Input: part model. Units: mm. Frame: model coordinates. A direction names the side the tool comes from. Coordinates: 2 decimals unless noted, no trailing zeros. Write each loop counter-clockwise with the first axis right and the second up, starting at its lowest first coordinate (ties: lowest second). Pieces come first, ordered by that corner, then holes. Notation, with made-up numbers: (47.25, 71.5) - (90.25, 71.5) arc R19 ccw to (90.25, 101.5) - close; hole circle Ø10 at (-29, 89.5). An arc over 180 degrees is marked (long way). Use a Markdown table: item, result. Add a question column.
Q1. Pin query (flat end, axial travel): P1, Ø2, axis at x = 10.16, z = 2.5, coming from the -Y side; P2, Ø1, axis at y = -9.5, z = 1.5, coming from the +X side. Return the tip coordinate at first contact, or that it passes through.
Q2. Section query A-A (z = 2.5). Return the cut outline in (x, y), then the cut area to 3 significant figures.
Q3. Section query D-D (x = 6.8). Return the cut outline in (y, z), then the cut area to 3 significant figures.
Q4. Mould query, pull axis Y, two halves, no side actions, for faces 6 (the face through (8, -25, 2)), 7 (the face through (8, -4, 1)), 8 (the face through (3.6, -14.3, 5)), 9 (the face through (5, 0, 2)). Classes: released by +Y, released by -Y, zero draft, split by the parting line, or undercut.
Q5. Material intervals for probe 1 along Y at (x, z) = (7, 0.4); probe 2 along Z at (x, y) = (10.16, -27.6); probe 3 along X at (y, z) = (-6.5, 4), sorted ascending. Write a range as from..to.
Q6. Set-up query: faces 1 (the face through (4, -14, 2)), 2 (the face through (9.6, -2, 2)), 3 (the face through (8.54, -27.03, 1.99)), 4 (the face through (6, -29, 2)), 5 (the face through (8.5, -2.03, 2.43)). Return all of +Z, -Z, +X, -X, +Y, -Y with unobstructed straight access to the full face (end or side cutting, diameter ignored); none if empty.
Q7. Section query B-B (x = 10.16). Return the cut outline in (y, z).
Q8. Section query C-C (y = -25.75). Return the cut outline in (x, z), then the cut area to 3 significant figures.
from build123d import *

# Parameters (mm, degrees)
RESSALTO_EXTRUS_O1_DEPTH    = 5
FURO_COM_FOLGA_DE_M32_D     = 3.4
FURO_COM_FOLGA_DE_M32_DEPTH = 4
FURO_COM_FOLGA_DE_M31_D     = 3.4
FURO_COM_FOLGA_DE_M31_DEPTH = 11.25
FURO_COM_FOLGA_DE_M31_TIP   = 1.021463052


with BuildPart() as part:
    # Esboço1 → Ressalto-extrusão1 (new body)
    with BuildSketch(Plane.XY):
        Polygon((12.7, -29), (0, -29), (0, 0), (9.6, 0), (9.6, -4), (4, -4), (4, -25), (12.7, -25), align=None)
    extrude(amount=RESSALTO_EXTRUS_O1_DEPTH)

    # Furo com folga de M32
    with Locations(Plane(origin=(0, -25, 0), x_dir=(1, 0, 0), z_dir=(0, 1, 0))):
        with Locations((10.16, -2.5)):
            Hole(FURO_COM_FOLGA_DE_M32_D / 2, depth=FURO_COM_FOLGA_DE_M32_DEPTH)

    # Furo com folga de M31
    with Locations(Plane(origin=(0, 0, 0), x_dir=(1, 0, 0), z_dir=(0, 1, 0))):
        with Locations((6.8, -2.5)):
            Hole(FURO_COM_FOLGA_DE_M31_D / 2, depth=FURO_COM_FOLGA_DE_M31_DEPTH)
            with Locations((0, 0, -(FURO_COM_FOLGA_DE_M31_DEPTH + FURO_COM_FOLGA_DE_M31_TIP / 2))):  # 118° drill point
                Cone(0, FURO_COM_FOLGA_DE_M31_D / 2, FURO_COM_FOLGA_DE_M31_TIP, mode=Mode.SUBTRACT)


solid = part.part
Values follow:
| question | item | result |
|---|---|---|
| 1 | P1 | y = -4 |
| 1 | P2 | x = 4 |
| 2 | outline | (0, -29) - (8.46, -29) - (8.46, -25) - (4, -25) - (4, -4) - (5.1, -4) - (5.1, 0) - (0, 0) - close; (8.5, -4) - (9.6, -4) - (9.6, 0) - (8.5, 0) - close; (11.86, -29) - (12.7, -29) - (12.7, -25) - (11.86, -25) - close |
| 2 | area | 146 mm2 |
| 3 | outline | (-29, 0) - (-25, 0) - (-25, 5) - (-29, 5) - close; (-4, 0) - (0, 0) - (0, 0.8) - (-4, 0.8) - close; (-4, 4.2) - (0, 4.2) - (0, 5) - (-4, 5) - close |
| 3 | area | 26.4 mm2 |
| 4 | face 6 | undercut |
| 4 | face 7 | undercut |
| 4 | face 8 | zero draft |
| 4 | face 9 | released by +Y |
| 5 | probe 1 | -29..-25, -4..0 |
| 5 | probe 2 | 0..0.8, 4.2..5 |
| 5 | probe 3 | 0..4 |
| 6 | face 1 | +Z, -Z, +X |
| 6 | face 2 | +Z, -Z, +X, +Y |
| 6 | face 3 | -Y |
| 6 | face 4 | +Z, -Z, +X, -X, -Y |
| 6 | face 5 | +Y |
| 7 | outline | (-29, 0) - (-25, 0) - (-25, 0.8) - (-29, 0.8) - close; (-29, 4.2) - (-25, 4.2) - (-25, 5) - (-29, 5) - close |
| 8 | outline | (0, 0) - (12.7, 0) - (12.7, 5) - (0, 5) - close; hole circle Ø3.4 at (10.16, 2.5) |
| 8 | area | 54.4 mm2 |
